from build123d import *

# Parameters (mm, degrees)
SKETCH_1_R          = 19
EXTRUDE_1_DEPTH     = 25
SKETCH_2_R          = 10
CUT_EXTRUDE_1_DEPTH = 5
SKETCH_3_R          = 3
CUT_EXTRUDE_2_DEPTH = 15
CUT_EXTRUDE_3_REACH = 21
SKETCH_4_R          = 1.1
FILLET_1_R          = 7


with BuildPart() as part:
    # 草圖1 → 填料-伸長1 (new body)
    with BuildSketch(Plane.XY):
        Circle(SKETCH_1_R)
    extrude(amount=EXTRUDE_1_DEPTH)

    # 草圖2 → 除料-伸長1 (cut)
    with BuildSketch(Plane(origin=(0, 0, 0), x_dir=(-1, 0, 0), z_dir=(0, 0, -1))):
        Circle(SKETCH_2_R)
    extrude(amount=-CUT_EXTRUDE_1_DEPTH, mode=Mode.SUBTRACT)

    # 草圖3 → 除料-伸長2 (cut)
    with BuildSketch(Plane(origin=(0, 0, 5), x_dir=(-1, 0, 0), z_dir=(0, 0, -1))):
        Circle(SKETCH_3_R)
    extrude(amount=-CUT_EXTRUDE_2_DEPTH, mode=Mode.SUBTRACT)

    # 草圖4 → 除料-伸長3 (cut, up to next)
    with BuildSketch(Plane(origin=(0, 0, 0), x_dir=(1, 0, 0), z_dir=(0, 1, 0)), mode=Mode.PRIVATE) as cut_extrude_3_sk1:
        with Locations((0, -10)):
            Circle(SKETCH_4_R)
    cut_extrude_3_tool1 = extrude(cut_extrude_3_sk1.sketch, amount=-CUT_EXTRUDE_3_REACH, mode=Mode.PRIVATE) & part.part
    add(cut_extrude_3_tool1.solids().sort_by_distance((0, 0, 10))[0], mode=Mode.SUBTRACT)

    # 圓角1
    fillet_1_edges = [part.edges().sort_by_distance(p)[0] for p in [
        (-19, 0, 25),
    ]]
    fillet(fillet_1_edges, radius=FILLET_1_R)


solid = part.part
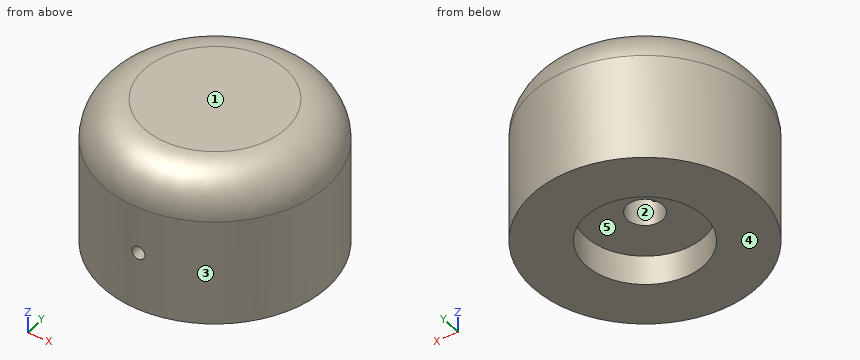
The model under review builds one solid part; all positions refer to its coordinate system, in mm. Face numbers are marked on the shaded views. A direction names the side the tool comes from. Round coordinates to 2 decimals unless told otherwise and drop trailing zeros. Loops run counter-clockwise (first coordinate to the right, second up) from the corner with the lowest first, then second, coordinate; pieces in that order, holes last. Notation, with made-up numbers: (82, 69) -> (127, 69) arc R17 cw to (127, 79) -> close; hole circle Ø6 at (1, -24). An arc over 180 degrees is marked (long way). Answer as CSV lines item,"result".
1) Add section A-A on x = 0. Write out the cut boundary in (y, z).
Geometry results:
outline,"(-19, 0) -> (-10, 0) -> (-10, 5) -> (-3, 5) -> (-3, 8.9) -> (-19, 8.9) -> close; (-19, 11.1) -> (-3, 11.1) -> (-3, 20) -> (3, 20) -> (3, 5) -> (10, 5) -> (10, 0) -> (19, 0) -> (19, 18) arc R7 ccw to (12, 25) -> (-12, 25) arc R7 ccw to (-19, 18) -> close"
2) Add section B-B on z = 4. Write out the cut boundary in (x, y).
Geometry results:
outline,"circle Ø38 at (0, 0); hole circle Ø20 at (0, 0)"
3) Add section C-C on z = 17.25. Write out the cut boundary in (x, y), plus the area to 3 significant figures.
Geometry results:
outline,"circle Ø38 at (0, 0); hole circle Ø6 at (0, 0)"
area,"1,110 mm²"
4) For P1, Ø2, axis at x = -2, z = 5.5, coming from the -Y side; P2, Ø8, axis at y = -14.5, z = 9, coming from the +X side; P3, Ø1, axis at y = 13.5, z = 15.5, coming from the -X side, all flat-tipped, find the tip position at first contact; note any pin that passes through.
Geometry results:
P1,"stops at y = -18.97"
P2,"stops at x = 15.84"
P3,"stops at x = -13.86"
5) Draft analysis for pull direction X (two halves, no side actions). For the marked faces 1, 2 and 3, state which applies: pulls with the +X half, pulls with the -X half, needs draft (parallel to the pull), parting line crosses it, or undercut.
Geometry results:
face 1,"needs draft"
face 2,"undercut"
face 3,"parting line crosses it"
6) To check wall thickness, follow line 1 along Y through (x, z) = (0, 3.25); line 2 along Z through (x, y) = (0, -7); line 3 along Z through (x, y) = (3.5, 2). State the ranges of each line that lie inside material, in increasing order. Write a range as from..to.
Geometry results:
line 1,"y = -19..-10, 10..19"
line 2,"z = 5..8.9, 11.1..25"
line 3,"z = 5..25"
7) Add section D-D on z = 10. Write out the cut boundary in (x, y).
Geometry results:
outline,"(-1.1, -18.97) -> (-1.1, -2.79) arc R3 cw (long way) to (1.1, -2.79) -> (1.1, -18.97) arc R19 ccw (long way) to start"
8) Tool access review of the marked faces 4 and 5: name each direction out of +Z, -Z, +X, -X, +Y, -Y from which nothing blocks a thin tool from reaching the whole face with its end or side.
Geometry results:
face 4,"-Z, +X, -X, +Y, -Y"
face 5,"-Z"
